Design review of the part shown in the three views and the two pictorial views. Dimensions are in mm from the part's minimum x, y and z. A direction names the side the tool comes from. Coordinates: 2 decimals unless noted, no trailing zeros. Loops run counter-clockwise (first coordinate to the right, second up) from the corner with the lowest first, then second, coordinate; pieces in that order, holes last. Notation, with made-up numbers: (71, 47.5) - (105, 47.5) arc R17 cw to (105, 53.5) - close; hole circle Ø1 at (-19.5, -22). An arc over 180 degrees is marked (long way). One line per item, written item: value. Start each with the question number.
1. For the marked faces 5 and 6, list the 3-axis set-ups (+Z, -Z, +X, -X, +Y, -Y) from which the entire face can be reached by the end or side of a thin tool; tool diameter is ignored.
2. Insertion check: pin 1 (3 mm diameter, centred on y = 61, z = 3, fed in from +X); pin 2 (10 mm diameter, centred on y = 72, z = 8.5, fed in from +X); pin 3 (4 mm diameter, centred on y = 47, z = 5, fed in from -X); pin 4 (6 mm diameter, centred on x = 51, y = 50, fed in from -Z). Each pin has a flat end and moves straight along its axis. Give the tip position at first contact, or say it passes through.
3. Take a section at D-D, the plane y = 90.5. State the section outline as (x, z) points (1 decimal), and give its area (3 significant figures).
4. Take a section at C-C, the plane x = 50.8. State the section outline as (y, z) points (1 decimal), and give its area (3 significant figures).
5. Take a section at B-B, the plane z = 11. State the section outline as (x, y) points (1 decimal).
6. The part is to be moulded in two halves that separate along Y. For the marked faces 1, 2, 3 and 4, say which applies: released by +Y, released by -Y, zero draft, split by the parting line, or undercut.
7. To check wall thickness, follow line 1 (Y direction, x = 50.8, z = 20); line 2 (Z direction, x = 45, y = 91); line 3 (X direction, y = 26.5, z = 5.75) (1 decimal). State the ranges of each line that lie inside material, in increasing order. Write a range as from..to.
8. Take a section at A-A, the plane y = 50.8. State the section outline as (x, z) points (1 decimal).
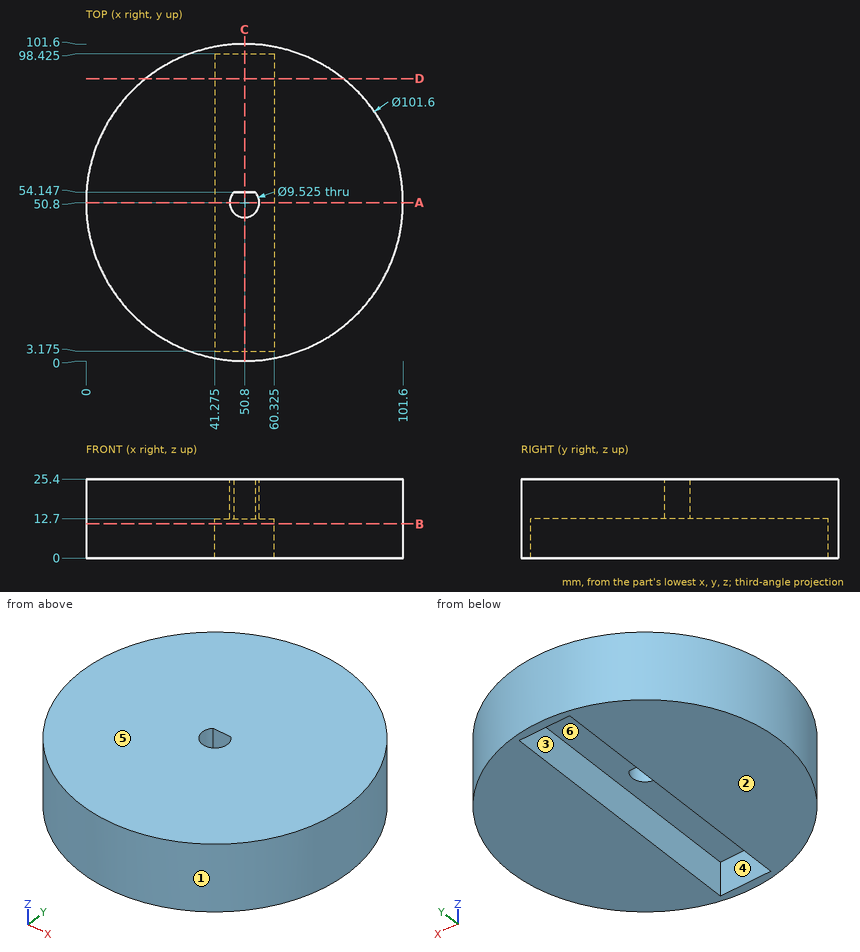
Solutions:
1. face 5: +Z, +X, -X, +Y, -Y
1. face 6: -Z
2. pin 1: x = 100.85
2. pin 2: x = 98.95
2. pin 3: x = 0.03
2. pin 4: through
3. outline: (19.1, 0) - (41.3, 0) - (41.3, 12.7) - (60.3, 12.7) - (60.3, 0) - (82.5, 0) - (82.5, 25.4) - (19.1, 25.4) - close
3. area: 1,370 mm2
4. outline: (0, 0) - (3.2, 0) - (3.2, 12.7) - (46, 12.7) - (46, 25.4) - (0, 25.4) - close; (54.1, 12.7) - (98.4, 12.7) - (98.4, 0) - (101.6, 0) - (101.6, 25.4) - (54.1, 25.4) - close
4. area: 1,270 mm2
5. outline: circle Ø101.6 at (50.8, 50.8); hole (41.3, 3.2) - (60.3, 3.2) - (60.3, 98.4) - (41.3, 98.4) - close
6. face 1: split by the parting line
6. face 2: zero draft
6. face 3: undercut
6. face 4: undercut
7. line 1: 0..46.04, 54.15..101.6
7. line 2: 12.7..25.4
7. line 3: 6.2..41.3, 60.3..95.4
8. outline: (0, 0) - (41.3, 0) - (41.3, 12.7) - (46, 12.7) - (46, 25.4) - (0, 25.4) - close; (55.6, 12.7) - (60.3, 12.7) - (60.3, 0) - (101.6, 0) - (101.6, 25.4) - (55.6, 25.4) - close
